Could you check a few things on this model? Use its own coordinates, in mm. A direction names the side the tool comes from. Round coordinates to 2 decimals unless told otherwise and drop trailing zeros. Write each loop counter-clockwise with the first axis right and the second up, starting at its lowest first coordinate (ties: lowest second). Pieces come first, ordered by that corner, then holes.
```python
from build123d import *

# Parameters (mm, degrees)
SKETCH1_R           = 4.572
BOSS_EXTRUDE1_DEPTH = 2.54
SKETCH2_R           = 2.413
BOSS_EXTRUDE2_DEPTH = 9.525
FILLET1_R           = 1.905
CUT_EXTRUDE1_DEPTH  = 1.905


with BuildPart() as part:
    # Sketch1 → Boss-Extrude1 (new body)
    with BuildSketch(Plane(origin=(0, 0, 0), x_dir=(0, 0, -1), z_dir=(1, 0, 0))):
        Circle(SKETCH1_R)
    extrude(amount=BOSS_EXTRUDE1_DEPTH)

    # Sketch2 → Boss-Extrude2 (add)
    with BuildSketch(Plane(origin=(2.54, 0, 0), x_dir=(0, 0, -1), z_dir=(1, 0, 0))):
        with Locations(Location((0, 0, 0), (0, 0, 180))):
            Circle(SKETCH2_R)
    extrude(amount=BOSS_EXTRUDE2_DEPTH)

    # Fillet1
    fillet1_edges = [part.edges().sort_by_distance(p)[0] for p in [
        (0, 0, 4.572),
    ]]
    fillet(fillet1_edges, radius=FILLET1_R)

    # Sketch3 → Cut-Extrude1 (cut)
    with BuildSketch(Plane.ZY):
        Polygon((1.573613406, -0.940185716), (1.601031418, 0.892696328), (0.027418011, 1.832882044), (-1.573613406, 0.940185716), (-1.601031418, -0.892696328), (-0.027418011, -1.832882044), align=None)
    extrude(amount=-CUT_EXTRUDE1_DEPTH, mode=Mode.SUBTRACT)


solid = part.part
```
Q1. I'm going to push flat-ended pins straight in: pin 1 Ø1 at (x, y) = (2.5, -2.5) entering from +Z; pin 2 Ø3 at (x, z) = (2, -2.5) entering from -Y; pin 3 Ø1 at (x, y) = (4.5, 2) entering from +Z. Where does each tip first touch, or does it pass through?
Q2. If I drill on L1, parallel to X at y = 2.25, z = -1; L2, parallel to X at y = 1, z = 1 (3 decimals); L3, parallel to Y at x = 1.25, z = -0.75, over which ranges is the centre line in solid material (lowest first)?
Q3. On a 3-axis mill with a long thin cutter (end or side, diameter ignored), from which of +Z, -Z, +X, -X, +Y, -Y can I reach the whole of each face in a straight line? I mean faces 5 (the flat face through (12.065, 0, 0)), 6 (the flat face through (1.905, 0, 0)), 7 (the cylindrical face through (7.236, 1.468, -1.915)). Say none if no direction works.
Q4. We'd pull the mould along Z, two halves only. Please class faces 1 (the flat face through (0.939, -1.393, 0.762)), 2 (the cylindrical face through (2.218, -4.463, 0.991)), 3 (the flat face through (2.54, -2, -2)), 4 (the flat face through (0.939, -1.356, -0.825)): pulls with the +Z half, pulls with the -Z half, needs draft (parallel to the pull), parting line crosses it, or undercut.
Q5. Imagine slicing it at B-B, the plane x = 6.25. Write out the boundary of the cut face in (y, z).
Q6. Imagine slicing it at A-A, the plane y = 0. Write out the boundary of the cut face in (x, z) (3 decimals).
Results found:
1. pin 1: stops at z = 4.11
1. pin 2: stops at y = -4.46
1. pin 3: stops at z = 1.89
2. L1: x = 0 to 2.54
2. L2: x = 1.905 to 12.065
2. L3: y = -4.39 to -1.4, 1.4 to 4.39
3. face 5: +Z, -Z, +X, +Y, -Y
3. face 6: -X
3. face 7: +X
4. face 1: undercut
4. face 2: parting line crosses it
4. face 3: needs draft
4. face 4: undercut
5. outline: circle Ø4.83 at (0, 0)
6. outline: (0, -2.667) arc R1.905 ccw to (1.905, -4.572) - (2.54, -4.572) - (2.54, -2.413) - (12.065, -2.413) - (12.065, 2.413) - (2.54, 2.413) - (2.54, 4.572) - (1.905, 4.572) arc R1.905 ccw to (0, 2.667) - (0, 1.588) - (1.905, 1.588) - (1.905, -1.588) - (0, -1.588) - close
